The listing builds one solid part. Answer for the finished solid, in the listing's coordinates (mm). Round coordinates to 2 decimals unless told otherwise and drop trailing zeros. Write each loop counter-clockwise with the first axis right and the second up, starting at its lowest first coordinate (ties: lowest second). Pieces come first, ordered by that corner, then holes.
Item 1: Find section B-B on y = 0.4. Give the number of separate pieces and of enclosed holes in the cut face, then the cut area to 3 significant figures.
Item 2: Each of these flat-tipped pins is pushed along its axis until it touches: pin 1 (3 mm diameter, centred on x = 39.5, z = 0, fed in from +Y); pin 2 (0.8 mm diameter, centred on x = 44, y = 0.5, fed in from -Z); pin 3 (0.8 mm diameter, centred on y = 0, z = -69, fed in from -X); pin 4 (0.8 mm diameter, centred on x = -43.5, y = 0, fed in from +Z). Where does it stop, or does it pass through?
Item 3: Find section A-A on z = 72. Give the vertices of the cut face in (x, y).
Item 4: Find the intervals of material crossed by probe 1 along X at (y, z) = (-0.05, 71); probe 2 along X at (y, z) = (-0.5, 5); probe 3 along Z at (x, y) = (-41, 0.55), in increasing order.
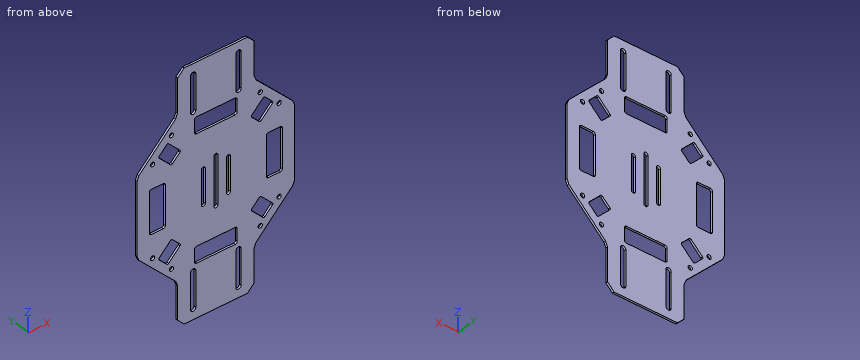
```python
from build123d import *

# Parameters (mm, degrees)
SKETCH1_R           = 1.6
BOSS_EXTRUDE1_DEPTH = 0.75


with BuildPart() as part:
    # Sketch1 → Boss-Extrude1 (new, symmetric)
    with BuildSketch(Plane.XZ):
        Polygon((-59, 26.610173055), (-59, -26.610173055), (-57.535533906, -30.145706961), (-30.164466094, -57.516774773), (-28.7, -61.052308679), (-28.7, -85.8), (-23.7, -90.8), (23.7, -90.8), (28.7, -85.8), (28.7, -61.052308679), (30.164466094, -57.516774773), (57.535533906, -30.145706961), (59, -26.610173055), (59, 26.610173055), (57.535533906, 30.145706961), (30.164466094, 57.516774773), (28.7, 61.052308679), (28.7, 85.8), (23.7, 90.8), (-23.7, 90.8), (-28.7, 85.8), (-28.7, 61.052308679), (-30.164466094, 57.516774773), (-57.535533906, 30.145706961), align=None)
        with Locations(Location((-33.234018716, -47.376154339, 0), (0, 0, 90))):
            Circle(SKETCH1_R, mode=Mode.SUBTRACT)
        with Locations(Location((-47.376154339, -33.234018716, 0), (0, 0, 90))):
            Circle(SKETCH1_R, mode=Mode.SUBTRACT)
        with Locations(Location((-47.376154339, 33.234018716, 0), (0, 0, 90))):
            Circle(SKETCH1_R, mode=Mode.SUBTRACT)
        with Locations(Location((-33.234018716, 47.376154339, 0), (0, 0, 90))):
            Circle(SKETCH1_R, mode=Mode.SUBTRACT)
        with Locations(Location((33.234018716, 47.376154339, 0), (0, 0, 90))):
            Circle(SKETCH1_R, mode=Mode.SUBTRACT)
        with Locations(Location((47.376154339, 33.234018716, 0), (0, 0, 90))):
            Circle(SKETCH1_R, mode=Mode.SUBTRACT)
        with Locations(Location((47.376154339, -33.234018716, 0), (0, 0, 90))):
            Circle(SKETCH1_R, mode=Mode.SUBTRACT)
        with Locations(Location((33.234018716, -47.376154339, 0), (0, 0, 90))):
            Circle(SKETCH1_R, mode=Mode.SUBTRACT)
        with BuildLine():
            Line((-19, -82.8), (-19, -56.8))
            ThreePointArc((-19, -56.8), (-17, -54.8), (-15, -56.8))
            Line((-15, -56.8), (-15, -82.8))
            ThreePointArc((-15, -82.8), (-17, -84.8), (-19, -82.8))
        make_face(mode=Mode.SUBTRACT)
        with BuildLine():
            Line((19, 82.8), (19, 56.8))
            ThreePointArc((19, 56.8), (17, 54.8), (15, 56.8))
            Line((15, 56.8), (15, 82.8))
            ThreePointArc((15, 82.8), (17, 84.8), (19, 82.8))
        make_face(mode=Mode.SUBTRACT)
        with BuildLine():
            Line((-15, 82.8), (-15, 56.8))
            ThreePointArc((-15, 56.8), (-17, 54.8), (-19, 56.8))
            Line((-19, 56.8), (-19, 82.8))
            ThreePointArc((-19, 82.8), (-17, 84.8), (-15, 82.8))
        make_face(mode=Mode.SUBTRACT)
        with BuildLine():
            Line((-14.5, 51.9), (14.5, 51.9))
            ThreePointArc((14.5, 51.9), (15.560660172, 51.460660172), (16, 50.4))
            Line((16, 50.4), (16, 41.4))
            ThreePointArc((16, 41.4), (15.560660172, 40.339339828), (14.5, 39.9))
            Line((14.5, 39.9), (-14.5, 39.9))
            ThreePointArc((-14.5, 39.9), (-15.560660172, 40.339339828), (-16, 41.4))
            Line((-16, 41.4), (-16, 50.4))
            ThreePointArc((-16, 50.4), (-15.560660172, 51.460660172), (-14.5, 51.9))
        make_face(mode=Mode.SUBTRACT)
        with BuildLine():
            Line((16, -41.4), (16, -50.4))
            ThreePointArc((16, -50.4), (15.560660172, -51.460660172), (14.5, -51.9))
            Line((14.5, -51.9), (-14.5, -51.9))
            ThreePointArc((-14.5, -51.9), (-15.560660172, -51.460660172), (-16, -50.4))
            Line((-16, -50.4), (-16, -41.4))
            ThreePointArc((-16, -41.4), (-15.560660172, -40.339339828), (-14.5, -39.9))
            Line((-14.5, -39.9), (14.5, -39.9))
            ThreePointArc((14.5, -39.9), (15.560660172, -40.339339828), (16, -41.4))
        make_face(mode=Mode.SUBTRACT)
        with BuildLine():
            Line((19, -56.8), (19, -82.8))
            ThreePointArc((19, -82.8), (17, -84.8), (15, -82.8))
            Line((15, -82.8), (15, -56.8))
            ThreePointArc((15, -56.8), (17, -54.8), (19, -56.8))
        make_face(mode=Mode.SUBTRACT)
        with BuildLine():
            Line((-10.9, -12.5), (-10.9, 12.5))
            ThreePointArc((-10.9, 12.5), (-9.4, 14), (-7.9, 12.5))
            Line((-7.9, 12.5), (-7.9, -12.5))
            ThreePointArc((-7.9, -12.5), (-9.4, -14), (-10.9, -12.5))
        make_face(mode=Mode.SUBTRACT)
        with BuildLine():
            Line((10.9, 12.5), (10.9, -12.5))
            ThreePointArc((10.9, -12.5), (9.4, -14), (7.9, -12.5))
            Line((7.9, -12.5), (7.9, 12.5))
            ThreePointArc((7.9, 12.5), (9.4, 14), (10.9, 12.5))
        make_face(mode=Mode.SUBTRACT)
        with BuildLine():
            Line((-32.526911935, -26.870057685), (-26.870057685, -32.526911935))
            ThreePointArc((-26.870057685, -32.526911935), (-26.577164466, -33.234018716), (-26.870057685, -33.941125497))
            Line((-26.870057685, -33.941125497), (-35.355339059, -42.426406871))
            ThreePointArc((-35.355339059, -42.426406871), (-36.062445841, -42.71930009), (-36.769552622, -42.426406871))
            Line((-36.769552622, -42.426406871), (-42.426406871, -36.769552622))
            ThreePointArc((-42.426406871, -36.769552622), (-42.71930009, -36.062445841), (-42.426406871, -35.355339059))
            Line((-42.426406871, -35.355339059), (-33.941125497, -26.870057685))
            ThreePointArc((-33.941125497, -26.870057685), (-33.234018716, -26.577164466), (-32.526911935, -26.870057685))
        make_face(mode=Mode.SUBTRACT)
        with BuildLine():
            Line((-26.870057685, 32.526911935), (-32.526911935, 26.870057685))
            ThreePointArc((-32.526911935, 26.870057685), (-33.234018716, 26.577164466), (-33.941125497, 26.870057685))
            Line((-33.941125497, 26.870057685), (-42.426406871, 35.355339059))
            ThreePointArc((-42.426406871, 35.355339059), (-42.71930009, 36.062445841), (-42.426406871, 36.769552622))
            Line((-42.426406871, 36.769552622), (-36.769552622, 42.426406871))
            ThreePointArc((-36.769552622, 42.426406871), (-36.062445841, 42.71930009), (-35.355339059, 42.426406871))
            Line((-35.355339059, 42.426406871), (-26.870057685, 33.941125497))
            ThreePointArc((-26.870057685, 33.941125497), (-26.577164466, 33.234018716), (-26.870057685, 32.526911935))
        make_face(mode=Mode.SUBTRACT)
        with BuildLine():
            Line((48.35, -16), (39.35, -16))
            ThreePointArc((39.35, -16), (38.289339828, -15.560660172), (37.85, -14.5))
            Line((37.85, -14.5), (37.85, 14.5))
            ThreePointArc((37.85, 14.5), (38.289339828, 15.560660172), (39.35, 16))
            Line((39.35, 16), (48.35, 16))
            ThreePointArc((48.35, 16), (49.410660172, 15.560660172), (49.85, 14.5))
            Line((49.85, 14.5), (49.85, -14.5))
            ThreePointArc((49.85, -14.5), (49.410660172, -15.560660172), (48.35, -16))
        make_face(mode=Mode.SUBTRACT)
        with BuildLine():
            Line((-39.35, -16), (-48.35, -16))
            ThreePointArc((-48.35, -16), (-49.410660172, -15.560660172), (-49.85, -14.5))
            Line((-49.85, -14.5), (-49.85, 14.5))
            ThreePointArc((-49.85, 14.5), (-49.410660172, 15.560660172), (-48.35, 16))
            Line((-48.35, 16), (-39.35, 16))
            ThreePointArc((-39.35, 16), (-38.289339828, 15.560660172), (-37.85, 14.5))
            Line((-37.85, 14.5), (-37.85, -14.5))
            ThreePointArc((-37.85, -14.5), (-38.289339828, -15.560660172), (-39.35, -16))
        make_face(mode=Mode.SUBTRACT)
        with BuildLine():
            Line((26.870057685, -32.526911935), (32.526911935, -26.870057685))
            ThreePointArc((32.526911935, -26.870057685), (33.234018716, -26.577164466), (33.941125497, -26.870057685))
            Line((33.941125497, -26.870057685), (42.426406871, -35.355339059))
            ThreePointArc((42.426406871, -35.355339059), (42.71930009, -36.062445841), (42.426406871, -36.769552622))
            Line((42.426406871, -36.769552622), (36.769552622, -42.426406871))
            ThreePointArc((36.769552622, -42.426406871), (36.062445841, -42.71930009), (35.355339059, -42.426406871))
            Line((35.355339059, -42.426406871), (26.870057685, -33.941125497))
            ThreePointArc((26.870057685, -33.941125497), (26.577164466, -33.234018716), (26.870057685, -32.526911935))
        make_face(mode=Mode.SUBTRACT)
        with BuildLine():
            Line((32.526911935, 26.870057685), (26.870057685, 32.526911935))
            ThreePointArc((26.870057685, 32.526911935), (26.577164466, 33.234018716), (26.870057685, 33.941125497))
            Line((26.870057685, 33.941125497), (35.355339059, 42.426406871))
            ThreePointArc((35.355339059, 42.426406871), (36.062445841, 42.71930009), (36.769552622, 42.426406871))
            Line((36.769552622, 42.426406871), (42.426406871, 36.769552622))
            ThreePointArc((42.426406871, 36.769552622), (42.71930009, 36.062445841), (42.426406871, 35.355339059))
            Line((42.426406871, 35.355339059), (33.941125497, 26.870057685))
            ThreePointArc((33.941125497, 26.870057685), (33.234018716, 26.577164466), (32.526911935, 26.870057685))
        make_face(mode=Mode.SUBTRACT)
        with BuildLine():
            Line((1.5, 17.75), (1.5, -17.75))
            ThreePointArc((1.5, -17.75), (0, -19.25), (-1.5, -17.75))
            Line((-1.5, -17.75), (-1.5, 17.75))
            ThreePointArc((-1.5, 17.75), (0, 19.25), (1.5, 17.75))
        make_face(mode=Mode.SUBTRACT)
    extrude(amount=BOSS_EXTRUDE1_DEPTH, both=True)


solid = part.part
```
Check values:
1. separate pieces: 1
1. enclosed holes: 23
1. area: 12,800 mm2
2. pin 1: passes through
2. pin 2: stops at z = -44.08
2. pin 3: stops at x = -28.7
2. pin 4: stops at z = 44.58
3. outline: (-28.7, -0.75) - (-19, -0.75) - (-19, 0.75) - (-28.7, 0.75) - close; (-15, -0.75) - (15, -0.75) - (15, 0.75) - (-15, 0.75) - close; (19, -0.75) - (28.7, -0.75) - (28.7, 0.75) - (19, 0.75) - close
4. probe 1: x = -28.7 to -19, -15 to 15, 19 to 28.7
4. probe 2: x = -59 to -49.85, -37.85 to -10.9, -7.9 to -1.5, 1.5 to 7.9, 10.9 to 37.85, 49.85 to 59
4. probe 3: z = -46.68 to -38.2, -33.93 to -16, 16 to 33.93, 38.2 to 46.68
